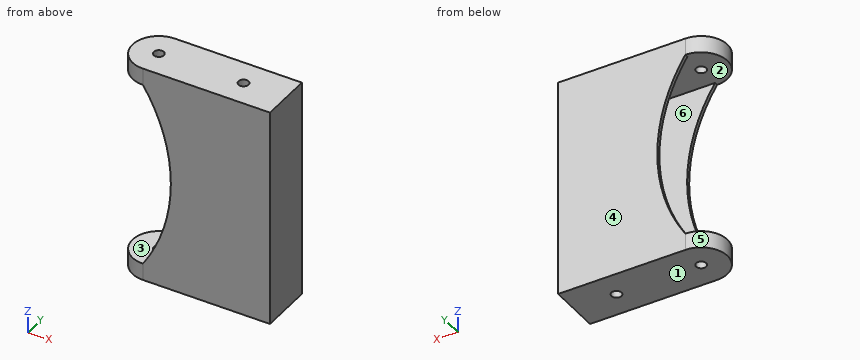
Autodesk Inventor part; units mm, degrees
ref_plane "YZ Plane" through (0, 0, 0) normal (1, 0, 0) x (0, 1, 0)
ref_plane "XZ Plane" through (0, 0, 0) normal (0, 1, 0) x (-1, 0, 0)
ref_plane "XY Plane" through (0, 0, 0) normal (0, 0, 1) x (1, 0, 0)
sketch "Sketch1" plane through (0, 0, 0) normal (0, 0, 1) x (1, 0, 0)
  circle A0 centre (0, 0) radius 3
  circle A1 centre (50, 0) radius 3
  line L0 (0, 15.5) -> (65, 15.5)
  line L1 (65, 15.5) -> (65, -15.5)
  line L2 (65, -15.5) -> (0, -15.5)
  arc A2 (0, 15.5) -> (0, -15.5) centre (0, 0) ccw
  dimension "d0" = 6
  dimension "d2" = 50
  dimension "d3" = 15
  dimension "d4" = 31
extrude "Extrusion1" add sketch "Sketch1" along normal blind 10
sketch "Sketch2" plane through (65, -15.5, 0) normal (1, 0, 0) x (0, 0, -1)
  line L0 (-10, 0) -> (120, 0)
  line L1 (120, 0) -> (120, 31)
  line L2 (120, 31) -> (-10, 31)
  line L3 (-10, 31) -> (-10, 0)
  point P0 (0, 15.5)
  dimension "d7" = 130
extrude "Extrusion2" add sketch "Sketch2" along normal blind 10
pattern_linear "Rectangular Pattern1" count 2 spacing 120 along (0, 0, -1) of "Extrusion1"
sketch "Sketch3" plane through (0, 15.5, 10) normal (0, 1, 0) x (1, 0, 0)
  line L0 (0, 10) -> (65, 10)
  line L1 (65, 120) -> (0, 120)
  line L2 (65, 120) -> (65, 10)
  arc A0 (0, 10) -> (0, 120) centre (-83.5165, 65) ccw
  dimension "d13" = 100
extrude "Extrusion3" add sketch "Sketch3" against normal blind 2
mirror "Mirror1" about plane through (0, 0, 0) normal (0, 1, 0) of "Extrusion3"
properties part number "FRONT"
Verification items for the finished model (mm, model axes). Face numbers are marked on the shaded views. A direction names the side the tool comes from. Coordinates: 2 decimals unless noted, no trailing zeros. Order: outer loops, then holes, each group sorted by start corner. A loop starts at its lowest first (then second) coordinate and runs counter-clockwise, first axis right, second up.
Item 1: Access from +Z, -Z, +X, -X, +Y, -Y to the whole of each face (thin tool, end or side, straight path). Record for the marked faces 5 and 6.
Filled in:
face 5: +Z, -Z, -X
face 6: -X
Item 2: Release check for a two-part mould opening along Z. For the marked faces 1, 2, 3 and 4 record: +Z half, -Z half, draft (parallel to the pull), parting line (faces both ways), or undercut.
Filled in:
face 1: -Z half
face 2: undercut
face 3: undercut
face 4: draft
Item 3: Depth check by flat-ended pin: pin 1 (1 mm diameter, centred on y = -11.5, z = -59, fed in from -X). Enter the tip coordinate at first touch or a pass-through.
Filled in:
pin 1: stops at x = 65
Item 4: Material ranges on L1, parallel to Y at x = 38, z = -44; L2, parallel to Z at x = -7, y = -10.5; L3, parallel to Y at x = 0, z = 7, recorded low to high.
Filled in:
L1: y = -15.5 to -13.5, 13.5 to 15.5
L2: z = -120 to -110, 0 to 10
L3: y = -15.5 to -3, 3 to 15.5
Item 5: Section check C-C, the plane z = -55. Enter the section's corners in (x, y), then the cut area to 3 significant figures.
Filled in:
outline: (16.48, -15.5) - (75, -15.5) - (75, 15.5) - (16.48, 15.5) - (16.48, 13.5) - (65, 13.5) - (65, -13.5) - (16.48, -13.5) - close
area: 504 mm2
Item 6: Section check A-A, the plane x = 59. Enter the section's corners in (y, z).
Filled in:
outline: (-15.5, -120) - (15.5, -120) - (15.5, 10) - (-15.5, 10) - close; hole (-13.5, -110) - (13.5, -110) - (13.5, 0) - (-13.5, 0) - close
Item 7: Section check D-D, the plane y = -10.5. Enter the section's corners in (x, z), then the cut area to 3 significant figures.
Filled in:
outline: (-11.4, -120) - (75, -120) - (75, 10) - (-11.4, 10) - (-11.4, 0) - (65, 0) - (65, -110) - (-11.4, -110) - close
area: 2,830 mm2
Item 8: Section check B-B, the plane y = 0. Enter the section's corners in (x, z).
Filled in:
outline: (-15.5, -120) - (-3, -120) - (-3, -110) - (-15.5, -110) - close; (-15.5, 0) - (-3, 0) - (-3, 10) - (-15.5, 10) - close; (3, -120) - (47, -120) - (47, -110) - (3, -110) - close; (3, 0) - (47, 0) - (47, 10) - (3, 10) - close; (53, -120) - (75, -120) - (75, 10) - (53, 10) - (53, 0) - (65, 0) - (65, -110) - (53, -110) - close
